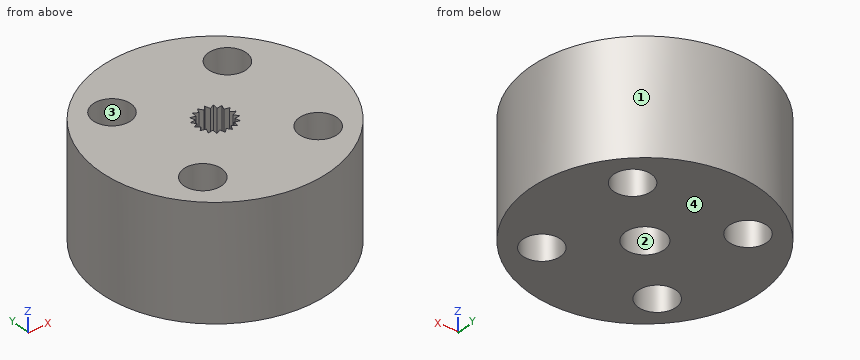
from build123d import *

# Parameters (mm, degrees)
F0_R      = 13.86
F1_DEPTH  = 13.77
F2_R      = 2.35
F2_R_2    = 2.275
F3_DEPTH  = 25
F4_R      = 2.35
F5_DEPTH  = 6.9
F7_R      = 2.38
F8_DEPTH  = 4.35
F9_DEPTH  = 5
F10_R     = 1.15
F11_DEPTH = 25
F12_R     = 2.35
F13_DEPTH = 25
F14_R     = 2.35
F15_DEPTH = 0.5
F16_R     = 1.15
F17_DEPTH = 25


with BuildPart() as f1:
    # F0 (on Top) → F1 (new body)
    with BuildSketch(Plane.XY):
        with Locations((0, 2.4059718373)):
            Circle(F0_R)
    extrude(amount=F1_DEPTH)

    # F2 (on face) → F3 (cut)
    with BuildSketch(Plane.XY.offset(13.77)):
        with Locations((0, 2.4059718373)):
            Circle(F2_R)
        with Locations((6.875, 9.2809718373)):
            Circle(F2_R_2)
        with Locations((-6.875, 9.2809718373)):
            Circle(F2_R_2)
        with Locations((-6.875, -4.4690281627)):
            Circle(F2_R_2)
        with Locations((6.875, -4.4690281627)):
            Circle(F2_R_2)
    extrude(amount=-F3_DEPTH, mode=Mode.SUBTRACT)

    # F4 (on face) → F5 (join)
    with BuildSketch(Plane.XY.offset(13.77)):
        with Locations((0, 2.4059718373)):
            Circle(F4_R)
    extrude(amount=-F5_DEPTH)

    # F7 (on face) → F8 (cut)
    with BuildSketch(Plane.XY.offset(13.77)):
        with Locations((0, 2.4059718373)):
            Circle(F7_R)
    extrude(amount=-F8_DEPTH, mode=Mode.SUBTRACT)

    # F6 (on face) → F9 (join)
    with BuildSketch(Plane.XY.offset(13.77)):
        with BuildLine():
            Line((1.2906450855, 3.7332204924), (1.9303061005, 3.7982068599))
            ThreePointArc((1.9303061005, 3.7982068599), (1.6592213389, 4.1122498183), (1.3377219765, 4.3744483836))
            Line((1.3377219765, 4.3744483836), (1.2906450855, 3.7332204924))
        make_face()
        with BuildLine():
            Line((1.6667554382, 3.2117509874), (2.2900668205, 3.0540412453))
            ThreePointArc((2.2900668205, 3.0540412453), (2.142739488, 3.4418615449), (1.9303061005, 3.7982068599))
            Line((1.9303061005, 3.7982068599), (1.6667554382, 3.2117509874))
        make_face()
        with BuildLine():
            ThreePointArc((2.3736116842, 2.2317088956), (2.3784023848, 2.3187818387), (2.38, 2.4059718373))
            ThreePointArc((2.38, 2.4059718373), (2.3574094927, 2.7331116906), (2.2900668205, 3.0540412453))
            Line((2.2900668205, 3.0540412453), (1.8418304863, 2.5930926248))
            Line((1.8418304863, 2.5930926248), (2.3736116842, 2.2317088956))
        make_face()
        with BuildLine():
            ThreePointArc((2.1708639479, 1.4303952285), (2.3072907469, 1.8221829978), (2.3736116842, 2.2317088956))
            Line((2.3736116842, 2.2317088956), (1.7947535953, 1.9518647336))
            Line((1.7947535953, 1.9518647336), (2.1708639479, 1.4303952285))
        make_face()
        with BuildLine():
            ThreePointArc((1.706277981, 0.7467504984), (1.9684765464, 1.0682498608), (2.1708639479, 1.4303952285))
            Line((2.1708639479, 1.4303952285), (1.5312029329, 1.365408861))
            Line((1.5312029329, 1.365408861), (1.706277981, 0.7467504984))
        make_face()
        with BuildLine():
            ThreePointArc((1.0358897076, 0.2632323492), (1.3922350227, 0.4756657368), (1.706277981, 0.7467504984))
            Line((1.706277981, 0.7467504984), (1.0829665987, 0.9044602404))
            Line((1.0829665987, 0.9044602404), (1.0358897076, 0.2632323492))
        make_face()
        with BuildLine():
            ThreePointArc((0.2405578474, 0.0381602058), (0.648069408, 0.1159050168), (1.0358897076, 0.2632323492))
            Line((1.0358897076, 0.2632323492), (0.5041085098, 0.6246160784))
            Line((0.5041085098, 0.6246160784), (0.2405578474, 0.0381602058))
        make_face()
        with BuildLine():
            ThreePointArc((-0.5837888395, 0.0986810903), (-0.1742629417, 0.0323601531), (0.2405578474, 0.0381602058))
            Line((0.2405578474, 0.0381602058), (-0.1355525053, 0.5596297109))
            Line((-0.1355525053, 0.5596297109), (-0.5837888395, 0.0986810903))
        make_face()
        with BuildLine():
            ThreePointArc((-1.3377219765, 0.4374952909), (-0.9755766088, 0.2351078894), (-0.5837888395, 0.0986810903))
            Line((-0.5837888395, 0.0986810903), (-0.7588638876, 0.717339453))
            Line((-0.7588638876, 0.717339453), (-1.3377219765, 0.4374952909))
        make_face()
        with BuildLine():
            ThreePointArc((-1.9303061005, 1.0137368146), (-1.6592213389, 0.6996938563), (-1.3377219765, 0.4374952909))
            Line((-1.3377219765, 0.4374952909), (-1.2906450855, 1.0787231821))
            Line((-1.2906450855, 1.0787231821), (-1.9303061005, 1.0137368146))
        make_face()
        with BuildLine():
            ThreePointArc((-2.2900668205, 1.7579024293), (-2.142739488, 1.3700821296), (-1.9303061005, 1.0137368146))
            Line((-1.9303061005, 1.0137368146), (-1.6667554382, 1.6001926872))
            Line((-1.6667554382, 1.6001926872), (-2.2900668205, 1.7579024293))
        make_face()
        with BuildLine():
            Line((-1.8418304863, 2.2188510498), (-2.3736116842, 2.580234779))
            ThreePointArc((-2.3736116842, 2.580234779), (-2.3678116315, 2.1654139899), (-2.2900668205, 1.7579024293))
            Line((-2.2900668205, 1.7579024293), (-1.8418304863, 2.2188510498))
        make_face()
        with BuildLine():
            Line((-1.7947535953, 2.860078941), (-2.1708639479, 3.3815484461))
            ThreePointArc((-2.1708639479, 3.3815484461), (-2.3072907469, 2.9897606768), (-2.3736116842, 2.580234779))
            Line((-2.3736116842, 2.580234779), (-1.7947535953, 2.860078941))
        make_face()
        with BuildLine():
            Line((-1.5312029329, 3.4465348136), (-1.706277981, 4.0651931762))
            ThreePointArc((-1.706277981, 4.0651931762), (-1.9684765464, 3.7436938138), (-2.1708639479, 3.3815484461))
            Line((-2.1708639479, 3.3815484461), (-1.5312029329, 3.4465348136))
        make_face()
        with BuildLine():
            Line((-1.0829665987, 3.9074834341), (-1.0358897076, 4.5487113253))
            ThreePointArc((-1.0358897076, 4.5487113253), (-1.3922350227, 4.3362779378), (-1.706277981, 4.0651931762))
            Line((-1.706277981, 4.0651931762), (-1.0829665987, 3.9074834341))
        make_face()
        with BuildLine():
            Line((-0.5041085098, 4.1873275962), (-0.2405578474, 4.7737834687))
            ThreePointArc((-0.2405578474, 4.7737834687), (-0.648069408, 4.6960386578), (-1.0358897076, 4.5487113253))
            Line((-1.0358897076, 4.5487113253), (-0.5041085098, 4.1873275962))
        make_face()
        with BuildLine():
            Line((0.1355525053, 4.2523139637), (0.5837888395, 4.7132625842))
            ThreePointArc((0.5837888395, 4.7132625842), (0.1742629417, 4.7795835214), (-0.2405578474, 4.7737834687))
            Line((-0.2405578474, 4.7737834687), (0.1355525053, 4.2523139637))
        make_face()
        with BuildLine():
            Line((0.7588638876, 4.0946042216), (1.3377219765, 4.3744483836))
            ThreePointArc((1.3377219765, 4.3744483836), (0.9755766088, 4.5768357852), (0.5837888395, 4.7132625842))
            Line((0.5837888395, 4.7132625842), (0.7588638876, 4.0946042216))
        make_face()
    extrude(amount=-F9_DEPTH)

    # F10 (on face) → F11 (cut)
    with BuildSketch(Plane(origin=(0, 0, 6.87), x_dir=(1, 0, 0), z_dir=(0, 0, -1))):
        with Locations((0, -2.4059718373)):
            Circle(F10_R)
    extrude(amount=-F11_DEPTH, mode=Mode.SUBTRACT)

    # F12 (on face) → F13 (cut)
    with BuildSketch(Plane.XY.offset(9.42)):
        with Locations((0, 2.4059718373)):
            Circle(F12_R)
    extrude(amount=-F13_DEPTH, mode=Mode.SUBTRACT)

    # F14 (on face) → F15 (join)
    with BuildSketch(Plane(origin=(0, 0, 9.42), x_dir=(1, 0, 0), z_dir=(0, 0, -1))):
        with Locations((0, -2.4059718373)):
            Circle(F14_R)
    extrude(amount=F15_DEPTH)

    # F16 (on face) → F17 (cut)
    with BuildSketch(Plane(origin=(0, 0, 8.92), x_dir=(1, 0, 0), z_dir=(0, 0, -1))):
        with Locations((0, -2.4059718373)):
            Circle(F16_R)
    extrude(amount=-F17_DEPTH, mode=Mode.SUBTRACT)


solid = f1.part
Input: part model. Units: mm. Frame: model coordinates. Face numbers are marked on the shaded views. Coordinates: 2 decimals unless noted, no trailing zeros. Order: outer loops, then holes, each group sorted by start corner. A loop starts at its lowest first (then second) coordinate and runs counter-clockwise, first axis right, second up. Notation, with made-up numbers: M 51.5,60.5 L 64.5,60.5 A20 ccw 64.5,97.5 Z; hole C 13,47.5 d10. An arc over 180 degrees is marked long. Answer in a Markdown table with one row per item.
(1) Draft query along X for the marked faces 1, 2, 3 and 4. Return one class per face: pulls with the +X half, pulls with the -X half, needs draft (parallel to the pull), parting line crosses it, or undercut.
Numbers:
| item | result |
|---|---|
| face 1 | parting line crosses it |
| face 2 | undercut |
| face 3 | undercut |
| face 4 | needs draft |
(2) Contact query for flat-ended pins moving along their axis: pin 1 Ø7.5 at (x, y) = (-6.88, -4.47) entering from +Z; pin 2 Ø4 at (y, z) = (13, 4) entering from +X; pin 3 Ø2 at (y, z) = (-2.5, 3.5) entering from -X; pin 4 Ø2 at (x, z) = (-9.5, 3) entering from -Y. Output: stop coordinate, or through.
Numbers:
| item | result |
|---|---|
| pin 1 | stops at z = 13.77 |
| pin 2 | stops at x = 10.87 |
| pin 3 | stops at x = -13.3 |
| pin 4 | stops at y = -8.54 |
(3) Section query C-C, the plane x = 12. Output: boundary loops of the cut face in (y, z), plus the area to 3 significant figures.
Numbers:
| item | result |
|---|---|
| outline | M -4.53,0 L 9.34,0 L 9.34,13.77 L -4.53,13.77 Z |
| area | 191 mm^2 |
(4) Section query A-A, the plane y = -5.5. Output: boundary loops of the cut face in (x, z), plus the area to 3 significant figures.
Numbers:
| item | result |
|---|---|
| outline | M -11.38,0 L -8.9,0 L -8.9,13.77 L -11.38,13.77 Z; M -4.85,0 L 4.85,0 L 4.85,13.77 L -4.85,13.77 Z; M 8.9,0 L 11.38,0 L 11.38,13.77 L 8.9,13.77 Z |
| area | 202 mm^2 |
(5) Material intervals for line 1 (Y direction, x = 5, z = 11.25); line 2 (Y direction, x = 7.5, z = 11.75); line 3 (X direction, y = 9.25, z = 3), sorted ascending. Write a range as [from, to].
Numbers:
| item | result |
|---|---|
| line 1 | y = [-10.52, -5.76], [-3.18, 7.99], [10.57, 15.33] |
| line 2 | y = [-9.25, -6.66], [-2.28, 7.09], [11.47, 14.06] |
| line 3 | x = [-12.05, -9.15], [-4.6, 4.6], [9.15, 12.05] |
(6) Section query B-B, the plane z = 8. Output: boundary loops of the cut face in (x, y) (3 decimals).
Numbers:
| item | result |
|---|---|
| outline | C 0,2.406 d27.72; hole C -6.875,-4.469 d4.55; hole C -6.875,9.281 d4.55; hole C 0,2.406 d4.7; hole C 6.875,-4.469 d4.55; hole C 6.875,9.281 d4.55 |
(7) Section query D-D, the plane y = -0.5. Output: boundary loops of the cut face in (x, z), plus the area to 3 significant figures.
Numbers:
| item | result |
|---|---|
| outline | M -13.55,0 L 13.55,0 L 13.55,13.77 L -13.55,13.77 Z |
| area | 373 mm^2 |
